CAD build for the part. Positions are in the model's coordinates, mm. Face numbers are marked on the shaded views. A direction names the side the tool comes from. Give positions to 0.01 mm unless a question says otherwise; leave off trailing zeros. Order: outer loops, then holes, each group sorted by start corner. A loop starts at its lowest first (then second) coordinate and runs counter-clockwise, first axis right, second up.
Item 1: Band-saw the part on B-B on y = 34. Give the cut face in (x, z).
Item 2: Wall check: L1, parallel to Z at x = 55, y = 27; L2, parallel to X at y = 30, z = 13.75; L3, parallel to Y at x = 8, z = 12. Give the ranges that are in metal, low to high.
Item 3: Flat gauge pin, fed straight in: P1, Ø12, axis at x = 31, z = 10, coming from the +Y side. Where does the tip first touch, or does it go through?
Item 4: Which spindle directions (+Z, -Z, +X, -X, +Y, -Y) get a long thin tool onto all of the face, cutting with end or side? Do the marked faces 4 and 5. Say none if no direction does.
Item 5: Two-plate mould, pull along X, no slides. Class the marked faces 1, 2 and 3: released by +X, released by -X, zero draft, split by the parting line, or undercut.
Item 6: Band-saw the part on A-A on x = 32. Give the cut face in (y, z), plus the area to 3 significant figures.
Item 7: Band-saw the part on C-C on x = 26. Give the cut face in (y, z).
Item 8: Band-saw the part on D-D on x = 16. Give the cut face in (y, z).
```python
from build123d import *

# Parameters (mm, degrees)
EXTRUDE_933_DEPTH      = 20
SKETCH6_R              = 3
SKETCH6_R_2            = 1.5
CUT_EXTRUDE_1730_DEPTH = 70
SKETCH7_R              = 1.5
SKETCH7_R_2            = 4
CUT_EXTRUDE_2086_DEPTH = 55.5
FILLET1_R              = 10
FILLET2_R              = 2


with BuildPart() as part:
    # Sketch2 → Extrude 933 (new body)
    with BuildSketch(Plane.XY):
        Polygon((0, 0), (55.5, 0), (55.5, 37), (53.5, 37), (53.5, 2), (2, 2), (2, 37), (0, 37), align=None)
    extrude(amount=EXTRUDE_933_DEPTH)

    # Sketch6 → Cut-Extrude 1730 (cut)
    with BuildSketch(Plane(origin=(0, 0, 0), x_dir=(-1, 0, 0), z_dir=(0, -1, 0))):
        with Locations(Location((-27.75, -10, 0), (0, 0, 180))):
            Circle(SKETCH6_R)
        with Locations(Location((-32.699747468, -14.949747468, 0), (0, 0, 270))):
            Circle(SKETCH6_R_2)
        with Locations(Location((-32.699747468, -5.050252532, 0), (0, 0, 180))):
            Circle(SKETCH6_R_2)
        with Locations(Location((-42.599747468, -14.949747468, 0), (0, 0, 270))):
            Circle(SKETCH6_R_2)
        with Locations(Location((-42.599747468, -5.050252532, 0), (0, 0, 180))):
            Circle(SKETCH6_R_2)
        with Locations(Location((-12.900252532, -5.050252532, 0), (0, 0, 270))):
            Circle(SKETCH6_R_2)
        with Locations(Location((-22.800252532, -5.050252532, 0), (0, 0, 270))):
            Circle(SKETCH6_R_2)
        with Locations(Location((-22.800252532, -14.949747468, 0), (0, 0, 180))):
            Circle(SKETCH6_R_2)
        with Locations(Location((-12.900252532, -14.949747468, 0), (0, 0, 180))):
            Circle(SKETCH6_R_2)
    extrude(amount=-CUT_EXTRUDE_1730_DEPTH, mode=Mode.SUBTRACT)

    # Sketch7 → Cut-Extrude 2086 (cut)
    with BuildSketch(Plane.ZY):
        with Locations(Location((17, 27, 0), (0, 0, 270))):
            Circle(SKETCH7_R)
        with Locations(Location((14.949747468, 22.050252532, 0), (0, 0, 270))):
            Circle(SKETCH7_R)
        with Locations(Location((10, 20, 0), (0, 0, 270))):
            Circle(SKETCH7_R)
        with Locations(Location((5.050252532, 22.050252532, 0), (0, 0, 270))):
            Circle(SKETCH7_R)
        with Locations(Location((10, 34, 0), (0, 0, 270))):
            Circle(SKETCH7_R)
        with Locations(Location((3, 27, 0), (0, 0, 270))):
            Circle(SKETCH7_R)
        with Locations(Location((10, 27, 0), (0, 0, 270))):
            Circle(SKETCH7_R_2)
    extrude(amount=-CUT_EXTRUDE_2086_DEPTH, mode=Mode.SUBTRACT)

    # Fillet1
    fillet1_edges = [part.edges().sort_by_distance(p)[0] for p in [
        (54.5, 37, 20),
        (54.5, 37, 0),
        (1, 37, 0),
        (1, 37, 20),
    ]]
    fillet(fillet1_edges, radius=FILLET1_R - 0.0001)  # a hair under: the kernel refuses the full size

    # Fillet2
    fillet2_edges = [part.edges().sort_by_distance(p)[0] for p in [
        (2, 2, 10),
        (53.5, 2, 10),
        (55.5, 0, 10),
        (0, 0, 10),
    ]]
    fillet(fillet2_edges, radius=FILLET2_R)


solid = part.part
```
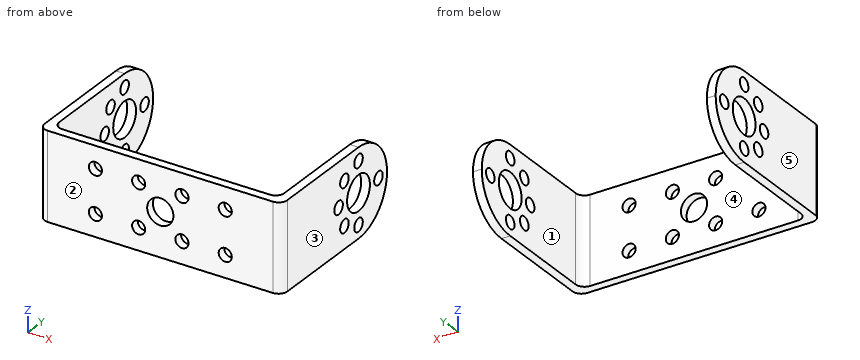
The answers:
1. outline: (0, 2.86) - (2, 2.86) - (2, 8.5) - (0, 8.5) - close; (0, 11.5) - (2, 11.5) - (2, 17.14) - (0, 17.14) - close; (53.5, 2.86) - (55.5, 2.86) - (55.5, 8.5) - (53.5, 8.5) - close; (53.5, 11.5) - (55.5, 11.5) - (55.5, 17.14) - (53.5, 17.14) - close
2. L1: z = 0 to 1.5, 4.5 to 6, 14 to 15.5, 18.5 to 20
2. L2: x = 0 to 2, 53.5 to 55.5
2. L3: y = 0 to 2
3. P1: stops at y = 2
4. face 4: +Z, -Z, +Y
4. face 5: +Z, -Z, -X, +Y, -Y
5. face 1: undercut
5. face 2: zero draft
5. face 3: released by +X
6. outline: (0, 0) - (2, 0) - (2, 3.72) - (0, 3.72) - close; (0, 6.38) - (2, 6.38) - (2, 13.62) - (0, 13.62) - close; (0, 16.28) - (2, 16.28) - (2, 20) - (0, 20) - close
6. area: 29.4 mm2
7. outline: (0, 0) - (2, 0) - (2, 7.56) - (0, 7.56) - close; (0, 12.44) - (2, 12.44) - (2, 20) - (0, 20) - close
8. outline: (0, 0) - (2, 0) - (2, 20) - (0, 20) - close
